Check sheet for the modelled part. Datum: model origin and axes. Units: mm. Face numbers are marked on the shaded views. Give positions to 0.01 mm unless a question says otherwise; leave off trailing zeros. Loops run counter-clockwise (first coordinate to the right, second up) from the corner with the lowest first, then second, coordinate; pieces in that order, holes last. Notation, with made-up numbers: (42, -25.75) -> (72, -25.75) arc R25 cw to (72, -4.75) -> close; hole circle Ø2 at (88.25, 76). An arc over 180 degrees is marked (long way). Write each question's results on one line, items separated by ' | '. Start each with the question number.
1. Material ranges on L1, parallel to X at y = 0, z = 1.85; L2, parallel to Y at x = -96.5, z = 2.4; L3, parallel to Y at x = 25.5, z = 5.25, recorded low to high. Write a range as from..to.
2. Cross-section at B-B on y = 0. Record the boundary of the cut face in (x, z).
3. Cross-section at A-A on x = -96.5. Record the boundary of the cut face in (y, z).
4. Cross-section at D-D on x = 69. Record the boundary of the cut face in (y, z), and give its area (3 significant figures).
5. Mould release check, pull along Y, two halves, no side actions. Record for the marked faces 1 and 2: +Y half, -Y half, draft (parallel to the pull), parting line (faces both ways), or undercut.
6. Gauge pin test, flat ends, axial feed: pin 1 Ø11 at (x, y) = (-96.5, 0) entering from -Z; pin 2 Ø1.8 at (x, z) = (-40.5, 2.5) entering from -Y; pin 3 Ø4.5 at (x, z) = (-24.5, 2.5) entering from +Y; pin 4 Ø9.5 at (x, y) = (-6, -2) entering from +Z. Record the tip position at first contact, or that the pin passes through.
7. Cross-section at C-C on z = 1.25. Record the boundary of the cut face in (x, y), and give its area (3 significant figures).
from build123d import *

# Parameters (mm, degrees)
F0_W     = 206
F0_H     = 36
F0_R     = 3.5
F1_DEPTH = 8
F2_W     = 19.0265765414
F2_H     = 3.3935653903
F3_DEPTH = 206.001
F5_DEPTH = 206.001


with BuildPart() as f1:
    # F0 (on Top) → F1 (new body)
    with BuildSketch(Plane.XY):
        Rectangle(F0_W, F0_H)
        with Locations((-96.5, 0)):
            Circle(F0_R, mode=Mode.SUBTRACT)
        with Locations((96.5, 0)):
            Circle(F0_R, mode=Mode.SUBTRACT)
    extrude(amount=F1_DEPTH)

    # F2 (on face) → F3 (cut, through all)
    with BuildSketch(Plane.YZ.offset(103)):
        with Locations((0.1401952468, 6.3032173049)):
            Rectangle(F2_W, F2_H)
    extrude(amount=-F3_DEPTH, mode=Mode.SUBTRACT)

    # F4 (on face) → F5 (cut, through all)
    with BuildSketch(Plane.YZ.offset(103)):
        Polygon((13.0982967094, 5.8882250451), (13.0982967094, 0), (18, 0), (18, 6.9697359577), align=None)
        Polygon((-13.0982967094, 5.8882250451), (-18, 6.9697359577), (-18, 0), (-13.0982967094, 0), align=None)
    extrude(amount=-F5_DEPTH, mode=Mode.SUBTRACT)


solid = f1.part
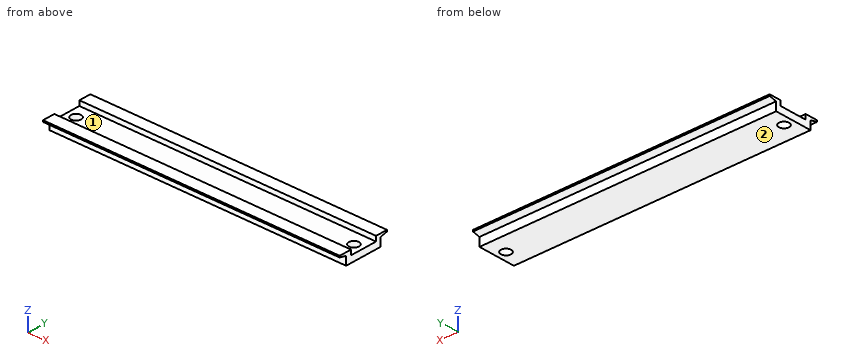
Geometry says:
1) L1: -103..-100, -93..93, 100..103 | L2: -13.1..-3.5, 3.5..13.1 | L3: -13.1..-9.37, 9.65..13.1
2) outline: (-103, 0) -> (-100, 0) -> (-100, 4.61) -> (-103, 4.61) -> close; (-93, 0) -> (93, 0) -> (93, 4.61) -> (-93, 4.61) -> close; (100, 0) -> (103, 0) -> (103, 4.61) -> (100, 4.61) -> close
3) outline: (-18, 6.97) -> (-13.1, 5.89) -> (-13.1, 0) -> (-3.5, 0) -> (-3.5, 4.61) -> (-9.37, 4.61) -> (-9.37, 8) -> (-18, 8) -> close; (3.5, 0) -> (13.1, 0) -> (13.1, 5.89) -> (18, 6.97) -> (18, 8) -> (9.65, 8) -> (9.65, 4.61) -> (3.5, 4.61) -> close
4) outline: (-18, 6.97) -> (-13.1, 5.89) -> (-13.1, 0) -> (13.1, 0) -> (13.1, 5.89) -> (18, 6.97) -> (18, 8) -> (9.65, 8) -> (9.65, 4.61) -> (-9.37, 4.61) -> (-9.37, 8) -> (-18, 8) -> close | area: 160 mm^2
5) face 1: undercut | face 2: draft
6) pin 1: z = 0 | pin 2: y = -13.1 | pin 3: y = 13.1 | pin 4: z = 4.61
7) outline: (-103, -13.1) -> (103, -13.1) -> (103, 13.1) -> (-103, 13.1) -> close; hole circle Ø7 at (-96.5, 0); hole circle Ø7 at (96.5, 0) | area: 5,320 mm^2
